Could you check a few things on this model? Use its own coordinates, in mm. Face numbers are marked on the shaded views. Coordinates: 2 decimals unless noted, no trailing zeros. Loops run counter-clockwise (first coordinate to the right, second up) from the corner with the lowest first, then second, coordinate; pieces in that order, holes last.
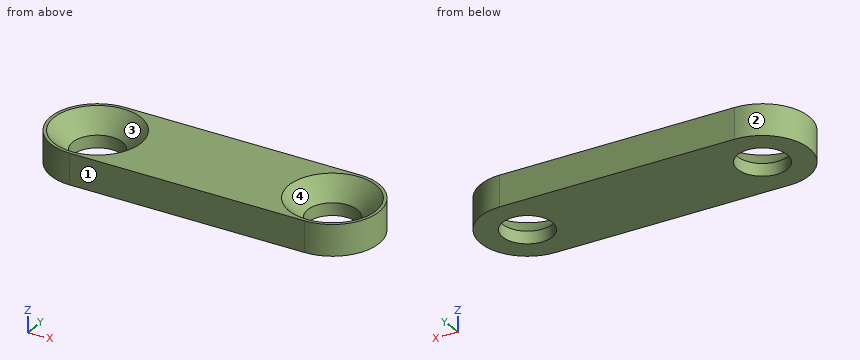
from build123d import *

# Parameters (mm, degrees)
EXTRUDE_1_DEPTH     = 2
SKETCH_2_R          = 1.6
CUT_EXTRUDE_1_DEPTH = 19.357559751
CHAMFER_1_SIZE      = 1.2


with BuildPart() as part:
    # 草图1 → 凸台-拉伸1 (new body)
    with BuildSketch(Plane.XY):
        with BuildLine():
            Line((0, -3), (-15, -3))
            ThreePointArc((-15, -3), (-18, 0), (-15, 3))
            Line((-15, 3), (0, 3))
            ThreePointArc((0, 3), (3, 0), (0, -3))
        make_face()
    extrude(amount=EXTRUDE_1_DEPTH)

    # 草图2 → 切除-拉伸1 (cut, through all)
    with BuildSketch(Plane.XY.offset(2)):
        Circle(SKETCH_2_R)
        with Locations((-15, 0)):
            Circle(SKETCH_2_R)
    extrude(amount=-CUT_EXTRUDE_1_DEPTH, mode=Mode.SUBTRACT)

    # 倒角1
    chamfer_1_edges = [part.edges().sort_by_distance(p)[0] for p in [
        (-1.6, 0, 2),
        (-16.6, 0, 2),
    ]]
    chamfer(chamfer_1_edges, length=CHAMFER_1_SIZE)


solid = part.part
(1) Imagine slicing it at B-B, the plane y = 0.3. State how many separate pieces and enclosed holes the cut face has, and give its area (3 significant figures).
Answers:
separate pieces: 3
enclosed holes: 0
area: 26.5 mm2
(2) We'd pull the mould along X, two halves only. Please class the marked faces 1, 2, 3 and 4: +X half, -X half, draft (parallel to the pull), parting line (faces both ways), or undercut.
Answers:
face 1: draft
face 2: -X half
face 3: undercut
face 4: undercut
(3) For pin 1 (2.5 mm diameter, centred on x = 0, y = 0, fed in from +Z), with a flat end and sliding along its axis, tell me the tip position at first contact or that it passes through.
Answers:
pin 1: passes through
(4) Imagine slicing it at A-A, the plane z = 1.6. Write out the boundary of the cut face in (x, y).
Answers:
outline: (-15, -3) - (0, -3) arc R3 ccw to (0, 3) - (-15, 3) arc R3 ccw to start; hole circle Ø4.8 at (-15, 0); hole circle Ø4.8 at (0, 0)
(5) Imagine slicing it at C-C, the plane z = 0.45. Write out the boundary of the cut face in (x, y).
Answers:
outline: (-15, -3) - (0, -3) arc R3 ccw to (0, 3) - (-15, 3) arc R3 ccw to start; hole circle Ø3.2 at (-15, 0); hole circle Ø3.2 at (0, 0)
(6) I need wall thicknesses on probe 1 along X at (y, z) = (-0.2, 0.6); probe 2 along X at (y, z) = (0.5, 1.3); probe 3 along Y at (x, z) = (-15, 0.25). Which ranges of each line are inside material? Lowest first, please.
Answers:
probe 1: x = -17.99 to -16.59, -13.41 to -1.59, 1.59 to 2.99
probe 2: x = -17.96 to -17.04, -12.96 to -2.04, 2.04 to 2.96
probe 3: y = -3 to -1.6, 1.6 to 3
